```python
from build123d import *

# Parameters (mm, degrees)
SKETCH2_R           = 1.25
BOSS_EXTRUDE1_DEPTH = 80
SKETCH3_R           = 1.25
BOSS_EXTRUDE2_DEPTH = 5
BOSS_EXTRUDE2_DRAFT = -5
CUT_EXTRUDE3_START  = -0.5
CUT_EXTRUDE3_DEPTH  = 0.5
LPATTERN1_COUNT     = 3
LPATTERN1_PITCH     = 1.5
CUT_EXTRUDE4_START  = -1.25
CUT_EXTRUDE4_DEPTH  = 0.5
LPATTERN2_COUNT     = 3
LPATTERN2_PITCH     = 1.5
SKETCH7_R           = 0.5
BOSS_EXTRUDE3_DEPTH = 26


with BuildPart() as part:
    # Sketch2 → Boss-Extrude1 (new body)
    with BuildSketch(Plane(origin=(0, 0, 0), x_dir=(1, 0, 0), z_dir=(0, 1, 0))):
        with Locations(Location((0, 0, 0), (0, 0, 270))):
            Circle(SKETCH2_R)
    extrude(amount=BOSS_EXTRUDE1_DEPTH)


with BuildPart() as boss_extrude2_tool:
    # Sketch3 → Boss-Extrude2 (with draft: the straight prism first)
    with BuildSketch(Plane.XZ):
        with Locations(Location((0, 0, 0), (0, 0, 270))):
            Circle(SKETCH3_R)
    extrude(amount=BOSS_EXTRUDE2_DEPTH)
    # Boss-Extrude2: the draft: its side faces are tilted about the plane it starts from
    boss_extrude2_sides = [boss_extrude2_tool.faces().sort_by_distance(p)[0] for p in [
        (0, -2.5, 1.25),
    ]]
    draft(boss_extrude2_sides, Plane.XZ, BOSS_EXTRUDE2_DRAFT)


with BuildPart() as part_1:
    add(part.part)

    # Boss-Extrude2: add boss_extrude2_tool
    add(boss_extrude2_tool.part)

    # Sketch4 → Cut-Extrude3 (cut)
    with BuildSketch(Plane.XZ.offset(5).offset(CUT_EXTRUDE3_START)):
        with BuildLine():
            Line((-0.87, 0.897552227), (-0.87, 1.445878608))
            ThreePointArc((-0.87, 1.445878608), (-1.687443318, 0), (-0.87, -1.445878608))
            Line((-0.87, -1.445878608), (-0.87, -0.897552227))
            ThreePointArc((-0.87, -0.897552227), (-1.25, 0), (-0.87, 0.897552227))
        make_face()
        with BuildLine():
            ThreePointArc((1.687443318, 0), (1.468935097, 0.830478556), (0.87, 1.445878608))
            Line((0.87, 1.445878608), (0.87, 0.897552227))
            ThreePointArc((0.87, 0.897552227), (1.151086443, 0.487339717), (1.25, 0))
            ThreePointArc((1.25, 0), (1.151086443, -0.487339717), (0.87, -0.897552227))
            Line((0.87, -0.897552227), (0.87, -1.445878608))
            ThreePointArc((0.87, -1.445878608), (1.468935097, -0.830478556), (1.687443318, 0))
        make_face()
    cut_extrude3 = extrude(amount=-CUT_EXTRUDE3_DEPTH, mode=Mode.SUBTRACT)

    # LPattern1: Cut-Extrude3 ×3
    with Locations(*[(0, i * LPATTERN1_PITCH, 0) for i in range(1, LPATTERN1_COUNT)]):
        add(cut_extrude3, mode=Mode.SUBTRACT)

    # Sketch6 → Cut-Extrude4 (cut)
    with BuildSketch(Plane.XZ.offset(5).offset(CUT_EXTRUDE4_START)):
        with BuildLine():
            Line((-1, 1.359214829), (-1, 0.75))
            ThreePointArc((-1, 0.75), (0, 1.25), (1, 0.75))
            Line((1, 0.75), (1, 1.359214829))
            ThreePointArc((1, 1.359214829), (0, 1.687443318), (-1, 1.359214829))
        make_face()
        with BuildLine():
            ThreePointArc((1, -0.75), (0, -1.25), (-1, -0.75))
            Line((-1, -0.75), (-1, -1.359214829))
            ThreePointArc((-1, -1.359214829), (0, -1.687443318), (1, -1.359214829))
            Line((1, -1.359214829), (1, -0.75))
        make_face()
    cut_extrude4 = extrude(amount=-CUT_EXTRUDE4_DEPTH, mode=Mode.SUBTRACT)

    # LPattern2: Cut-Extrude4 ×3
    with Locations(*[(0, i * LPATTERN2_PITCH, 0) for i in range(1, LPATTERN2_COUNT)]):
        add(cut_extrude4, mode=Mode.SUBTRACT)

    # Sketch7 → Boss-Extrude3 (add)
    with BuildSketch(Plane.XZ.offset(5)):
        with Locations(Location((0, 0, 0), (0, 0, 270))):
            Circle(SKETCH7_R)
    extrude(amount=BOSS_EXTRUDE3_DEPTH)


solid = part_1.part
```
The model under review builds one solid part; all positions refer to its coordinate system, in mm. A direction names the side the tool comes from. Round coordinates to 2 decimals unless told otherwise and drop trailing zeros. Loops run counter-clockwise (first coordinate to the right, second up) from the corner with the lowest first, then second, coordinate; pieces in that order, holes last.
Item 1: For faces 1 (the face through (-1, -5, 0)), 2 (the face through (-1.22, 39.44, -0.27)), 3 (the face through (0, 80, 0)), list the 3-axis set-ups (+Z, -Z, +X, -X, +Y, -Y) from which the entire face can be reached by the end or side of a thin tool; tool diameter is ignored.
Determined:
face 1: -Y
face 2: +Y
face 3: +Z, -Z, +X, -X, +Y
Item 2: Clearance check with flat-ended pins moving along their axes: pin 1 Ø1 at (x, y) = (-1.5, 61) entering from -Z; pin 2 Ø2 at (y, z) = (15.5, 0.5) entering from +X; pin 3 Ø0.5 at (x, z) = (-1, 0.5) entering from -Y. State where each tip first meets the part, or that it passes through.
Determined:
pin 1: stops at z = -0.75
pin 2: stops at x = 1.25
pin 3: stops at y = -5
Item 3: For line 1 (X direction, y = 44, z = -0.25); line 2 (Y direction, x = -0.3, z = -0.5); line 3 (X direction, y = -3.5, z = -0.2), list the stretches that pass through material, from the lowest coordinate up.
Determined:
line 1: x = -1.22 to 1.22
line 2: y = -5 to 80
line 3: x = -1.54 to 1.54
Item 4: Take a section at A-A (y = -18.5). Write out the cut boundary in (x, z), then the cut area to 3 significant figures.
Determined:
outline: circle Ø1 at (0, 0)
area: 0.785 mm2
Item 5: Take a section at B-B (y = 58). Write out the cut boundary in (x, z), then the cut area to 3 significant figures.
Determined:
outline: circle Ø2.5 at (0, 0)
area: 4.91 mm2
